Here's how the part is built. I have some questions about the finished solid (model axes, mm). A direction names the side the tool comes from. Give positions to 0.01 mm unless a question says otherwise; leave off trailing zeros. Loops run counter-clockwise (first coordinate to the right, second up) from the corner with the lowest first, then second, coordinate; pieces in that order, holes last. Notation, with made-up numbers: (59, -20) - (90, -20) arc R22 cw to (90, 4) - close; hole circle Ø7 at (79.25, 88). An arc over 180 degrees is marked (long way). Put each result on its own line as item: value. Start each with the question number.
from build123d import *

# Parameters (mm, degrees)
BOSS_EXTRUDE1_DEPTH     = 5
BOSS_EXTRUDE3_DEPTH     = 33
CUT_EXTRUDE2_DEPTH      = 121.706255016
CUT_EXTRUDE2_DEPTH_BACK = 121.706255016
SKETCH7_W               = 40
SKETCH7_H               = 23
CUT_EXTRUDE4_START      = 5
SKETCH3_W               = 80
SKETCH3_H               = 53
CUT_EXTRUDE4_DEPTH      = 4
SKETCH11_W              = 30
SKETCH11_H              = 0.5
SKETCH10_W              = 7
SKETCH10_H              = 0.5
BOSS_EXTRUDE4_START     = -54.5
BOSS_EXTRUDE4_DEPTH     = 20
BOSS_EXTRUDE5_DEPTH     = 20
BOSS_EXTRUDE6_DEPTH     = 10
CHAMFER1_SIZE           = 2


with BuildPart() as part:
    # Sketch1 → Boss-Extrude1 (new body)
    with BuildSketch(Plane(origin=(0, 0, 0), x_dir=(1, 0, 0), z_dir=(0, 1, 0))):
        with BuildLine():
            Line((-39.5, 40), (39.5, 40))
            ThreePointArc((39.5, 40), (50.106601718, 35.606601718), (54.5, 25))
            Line((54.5, 25), (54.5, -25))
            ThreePointArc((54.5, -25), (50.106601718, -35.606601718), (39.5, -40))
            Line((39.5, -40), (-39.5, -40))
            ThreePointArc((-39.5, -40), (-50.106601718, -35.606601718), (-54.5, -25))
            Line((-54.5, -25), (-54.5, 25))
            ThreePointArc((-54.5, 25), (-50.106601718, 35.606601718), (-39.5, 40))
        make_face()
    extrude(amount=BOSS_EXTRUDE1_DEPTH)

    # Sketch1<3> → Boss-Extrude3 (add)
    with BuildSketch(Plane(origin=(0, 0, 0), x_dir=(1, 0, 0), z_dir=(0, 1, 0))):
        with BuildLine():
            Line((-39.5, 40), (39.5, 40))
            ThreePointArc((39.5, 40), (50.106601718, 35.606601718), (54.5, 25))
            Line((54.5, 25), (54.5, -25))
            ThreePointArc((54.5, -25), (50.106601718, -35.606601718), (39.5, -40))
            Line((39.5, -40), (-39.5, -40))
            ThreePointArc((-39.5, -40), (-50.106601718, -35.606601718), (-54.5, -25))
            Line((-54.5, -25), (-54.5, 25))
            ThreePointArc((-54.5, 25), (-50.106601718, 35.606601718), (-39.5, 40))
        make_face()
        with BuildLine():
            ThreePointArc((-39.5, 33), (-45.156854249, 30.656854249), (-47.5, 25))
            Line((-47.5, 25), (-47.5, -25))
            ThreePointArc((-47.5, -25), (-45.156854249, -30.656854249), (-39.5, -33))
            Line((-39.5, -33), (39.5, -33))
            ThreePointArc((39.5, -33), (45.156854249, -30.656854249), (47.5, -25))
            Line((47.5, -25), (47.5, 25))
            ThreePointArc((47.5, 25), (45.156854249, 30.656854249), (39.5, 33))
            Line((39.5, 33), (-39.5, 33))
        make_face(mode=Mode.SUBTRACT)
    extrude(amount=BOSS_EXTRUDE3_DEPTH)

    # Sketch7 → Cut-Extrude2 (cut, two sides: drawn at the far end of the back side and taken through both)
    with BuildSketch(Plane.ZY.offset(54.5).offset(-CUT_EXTRUDE2_DEPTH_BACK)):
        with Locations((0, 16.5)):
            Rectangle(SKETCH7_W, SKETCH7_H)
    extrude(amount=CUT_EXTRUDE2_DEPTH + CUT_EXTRUDE2_DEPTH_BACK, mode=Mode.SUBTRACT)

    # Sketch3 → Cut-Extrude4 (cut)
    with BuildSketch(Plane(origin=(0, 0, 0), x_dir=(1, 0, 0), z_dir=(0, 1, 0)).offset(CUT_EXTRUDE4_START)):
        Rectangle(SKETCH3_W, SKETCH3_H)
    extrude(amount=-CUT_EXTRUDE4_DEPTH, mode=Mode.SUBTRACT)

    # Sweep2: sweep along a path in Sketch13
    with BuildLine(Plane(origin=(0, 0, 0), x_dir=(0, 0, -1), z_dir=(1, 0, 0))) as sweep2_path:
        Line((26.75, 5), (26.75, 8.08))
        Line((26.75, 8.08), (19.75, 8.08))
    # Sketch11 → Sweep2 (sweep)
    with BuildSketch(Plane(origin=(0, 5, 0), x_dir=(1, 0, 0), z_dir=(0, 1, 0))):
        with Locations((0, 26.75)):
            Rectangle(SKETCH11_W, SKETCH11_H)
    sweep(path=sweep2_path.line, transition=Transition.RIGHT)

    # Sweep3: sweep along a path in Sketch12
    with BuildLine(Plane(origin=(0, 0, 0), x_dir=(0, 0, -1), z_dir=(1, 0, 0))) as sweep3_path:
        Line((-26.75, 5), (-26.75, 8.08))
        Line((-26.75, 8.08), (-19.75, 8.08))
    # Sketch10 → Sweep3 (sweep)
    with BuildSketch(Plane(origin=(0, 5, 0), x_dir=(1, 0, 0), z_dir=(0, 1, 0))):
        with Locations((0, -26.75)):
            Rectangle(SKETCH10_W, SKETCH10_H)
    sweep(path=sweep3_path.line, transition=Transition.RIGHT)

    # Sketch19 → Boss-Extrude4 (add, symmetric)
    with BuildSketch(Plane(origin=(54.5, 0, 0), x_dir=(0, 0, -1), z_dir=(1, 0, 0)).offset(BOSS_EXTRUDE4_START)):
        Polygon((36.2, -1), (37.2, 0), (33, 0), (33, -2), (37.2, -2), align=None)
    boss_extrude4 = extrude(amount=BOSS_EXTRUDE4_DEPTH, both=True)

    # Mirror2: Boss-Extrude4 across plane
    add(boss_extrude4.mirror(Plane.XY))

    # Sketch20 → Boss-Extrude5 (add, symmetric)
    with BuildSketch(Plane.XY):
        Polygon((50.7, -1), (51.7, 0), (47.5, 0), (47.5, -2), (51.7, -2), align=None)
    boss_extrude5 = extrude(amount=BOSS_EXTRUDE5_DEPTH, both=True)

    # Mirror3: Boss-Extrude5 across plane
    add(boss_extrude5.mirror(Plane(origin=(0, 0, 0), x_dir=(0, 0, 1), z_dir=(1, 0, 0))))

    # Sketch21 → Boss-Extrude6 (add, symmetric)
    with BuildSketch(Plane(origin=(0, 0, 0), x_dir=(0, 0, -1), z_dir=(1, 0, 0))):
        Polygon((-36.2, 34), (-37.2, 33), (-33, 33), (-33, 35), (-37.2, 35), align=None)
    boss_extrude6 = extrude(amount=BOSS_EXTRUDE6_DEPTH, both=True)

    # Mirror4: Boss-Extrude6 across plane
    add(boss_extrude6.mirror(Plane.XY))

    # Chamfer1
    chamfer1_edges = [part.edges().sort_by_distance(p)[0] for p in [
        (-47.5, -2, 0),
        (0, -2, -33),
        (47.5, -2, 0),
        (0, -2, 33),
        (0, 35, -33),
        (0, 35, 33),
    ]]
    chamfer(chamfer1_edges, length=CHAMFER1_SIZE - 0.0001)  # a hair under: the kernel refuses the full size


solid = part.part
1) Suppose I cut it at A-A on z = -1. Give the number of separate pieces and of enclosed holes in the cut face, plus the area to 3 significant figures.
2) Suppose I cut it at C-C on y = 30. Please give me the cut outline in (x, z), plus the area to 3 significant figures.
3) Which directions (+Z, -Z, +X, -X, +Y, -Y) give clear straight access to the entire face, cutting with the end or side of a thin tool? Please do faces 4 (the cylindrical face through (-45.094, 18.804, -30.719)), 5 (the flat face through (-1, 3, 26.5)), 6 (the flat face through (-51, -2, 0)).
4) Thinking about a two-plate mould opening in X: for faces 1 (the flat face through (1, 16, 40)), 2 (the cylindrical face through (49.99, 16.27, -35.72)), 3 (the cylindrical face through (-45.219, 18.804, 30.594)), which applies, pulls with the +X half, pulls with the -X half, needs draft (parallel to the pull), parting line crosses it, or undercut?
5) Suppose I cut it at B-B on z = -22. Please give me the cut outline in (x, y).
6) I'm going to push flat-ended pins straight in: P1, Ø1, axis at x = -49.5, y = -1.5, coming from the -Z side; P2, Ø3, axis at x = 20.5, z = -14, coming from the +Y side; P3, Ø5, axis at y = 23, z = -26, coming from the -X side; P4, Ø7.5, axis at x = 4, z = -23, coming from the -Y side. Where does each tip first touch, or does it pass through?
7) I need wall thicknesses on line 1 (Z direction, x = 35, y = 10); line 2 (X direction, y = 10.5, z = 22.5); line 3 (Y direction, x = 16.5, z = 10). Which ranges of each line are inside material? Lowest first, please.
Ans:
1. separate pieces: 3
1. enclosed holes: 0
1. area: 306 mm²
2. outline: (-54.5, -25) arc R15 ccw to (-39.5, -40) - (39.5, -40) arc R15 ccw to (54.5, -25) - (54.5, 25) arc R15 ccw to (39.5, 40) - (-39.5, 40) arc R15 ccw to (-54.5, 25) - close; hole (-47.5, -25) arc R8 ccw to (-39.5, -33) - (39.5, -33) arc R8 ccw to (47.5, -25) - (47.5, 25) arc R8 ccw to (39.5, 33) - (-39.5, 33) arc R8 ccw to (-47.5, 25) - close
2. area: 2,310 mm²
3. face 4: +Y
3. face 5: none
3. face 6: +Z, -Z, +X, -X, -Y
4. face 1: needs draft
4. face 2: pulls with the +X half
4. face 3: undercut
5. outline: (-54.5, 0) - (54.5, 0) - (54.5, 33) - (47.5, 33) - (47.5, 5) - (40, 5) - (40, 1) - (-40, 1) - (-40, 5) - (-47.5, 5) - (-47.5, 33) - (-54.5, 33) - close; (-15, 7.83) - (15, 7.83) - (15, 8.33) - (-15, 8.33) - close
6. P1: stops at z = -20
6. P2: stops at y = 1
6. P3: stops at x = -54.5
6. P4: stops at y = 0
7. line 1: z = -40 to -33, 33 to 40
7. line 2: x = -54.5 to -47.5, 47.5 to 54.5
7. line 3: y = 0 to 1
